from build123d import *

# Parameters (mm, degrees)
SKETCH1_R           = 3.5
BOSS_EXTRUDE1_DEPTH = 4
SKETCH2_R           = 1.5
BOSS_EXTRUDE2_DEPTH = 8
CUT_EXTRUDE1_DEPTH  = 2
FILLET1_R           = 0.5


with BuildPart() as part:
    # Sketch1 → Boss-Extrude1 (new body)
    with BuildSketch(Plane(origin=(0, 0, 0), x_dir=(0, 0, -1), z_dir=(1, 0, 0))):
        Circle(SKETCH1_R)
    extrude(amount=BOSS_EXTRUDE1_DEPTH)

    # Sketch2 → Boss-Extrude2 (add)
    with BuildSketch(Plane(origin=(4, 0, 0), x_dir=(0, 0, -1), z_dir=(1, 0, 0))):
        Circle(SKETCH2_R)
    extrude(amount=BOSS_EXTRUDE2_DEPTH)

    # Sketch3 → Cut-Extrude1 (cut)
    with BuildSketch(Plane.ZY):
        Polygon((0, 1.732050808), (-1.5, 0.866025404), (-1.5, -0.866025404), (0, -1.732050808), (1.5, -0.866025404), (1.5, 0.866025404), align=None)
    extrude(amount=-CUT_EXTRUDE1_DEPTH, mode=Mode.SUBTRACT)

    # Fillet1
    fillet1_edges = [part.edges().sort_by_distance(p)[0] for p in [
        (0, 0, 3.5),
        (4, 0, 3.5),
    ]]
    fillet(fillet1_edges, radius=FILLET1_R)


solid = part.part
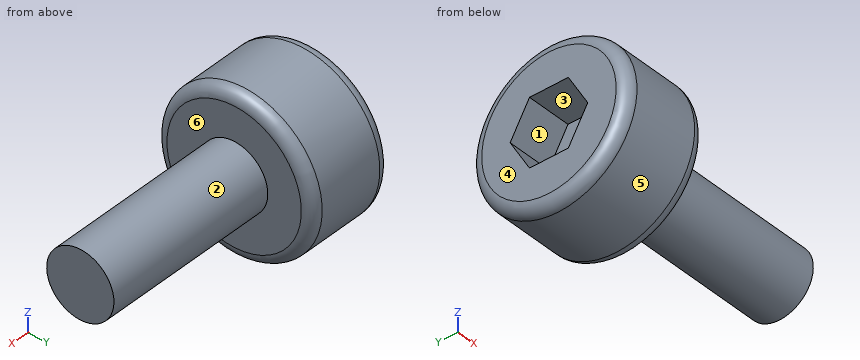
The model under review builds one solid part; all positions refer to its coordinate system, in mm. Face numbers are marked on the shaded views. A direction names the side the tool comes from. Coordinates: 2 decimals unless noted, no trailing zeros. Loops run counter-clockwise (first coordinate to the right, second up) from the corner with the lowest first, then second, coordinate; pieces in that order, holes last.
(1) Consider section A-A, the plane y = 0. Give the boundary of the cut face in (x, z), plus the area to 3 significant figures.
Determined:
outline: (0, -3) arc R0.5 ccw to (0.5, -3.5) - (3.5, -3.5) arc R0.5 ccw to (4, -3) - (4, -1.5) - (12, -1.5) - (12, 1.5) - (4, 1.5) - (4, 3) arc R0.5 ccw to (3.5, 3.5) - (0.5, 3.5) arc R0.5 ccw to (0, 3) - (0, 1.5) - (2, 1.5) - (2, -1.5) - (0, -1.5) - close
area: 45.8 mm2
(2) Tool access review of the marked faces 5 and 6: name each direction out of +Z, -Z, +X, -X, +Y, -Y from which nothing blocks a thin tool from reaching the whole face with its end or side.
Determined:
face 5: +X, -X
face 6: +X
(3) Consider section C-C, the plane x = 3.25. Give the boundary of the cut face in (y, z), plus the area to 3 significant figures.
Determined:
outline: circle Ø7 at (0, 0)
area: 38.5 mm2
(4) Draft analysis for pull direction Y (two halves, no side actions). For the marked faces 1, 2, 3 and 4, state which applies: +Y half, -Y half, draft (parallel to the pull), parting line (faces both ways), or undercut.
Determined:
face 1: undercut
face 2: parting line
face 3: undercut
face 4: draft
(5) Insertion check: P1, Ø2, axis at x = 7.5, y = -2, coming from the -Z side; P2, Ø1.5, axis at x = 4, z = -2, coming from the -Y side; P3, Ø0.5, axis at x = 1, y = -0.5, coming from the -Z side. Each pin has a flat end and moves straight along its axis. Give the tip position at first contact, or say it passes through.
Determined:
P1: stops at z = -1.12
P2: stops at y = -3.21
P3: stops at z = -3.49
(6) Consider section D-D, the plane x = 8.5. Give the boundary of the cut face in (y, z).
Determined:
outline: circle Ø3 at (0, 0)
(7) Wall thickness on L1, parallel to X at y = 2.25, z = -0.5; L2, parallel to Z at x = 1, y = 1.25; L3, parallel to X at y = -1, z = -0.5: over which ranges is each line inside the solid? List them lowest first.
Determined:
L1: x = 0 to 4
L2: z = -3.27 to -0.83, 0.83 to 3.27
L3: x = 2 to 12
(8) Consider section B-B, the plane x = 1.75. Give the boundary of the cut face in (y, z), plus the area to 3 significant figures.
Determined:
outline: circle Ø7 at (0, 0); hole (-1.73, 0) - (-0.87, -1.5) - (0.87, -1.5) - (1.73, 0) - (0.87, 1.5) - (-0.87, 1.5) - close
area: 30.7 mm2
